The model under review builds one solid part; all positions refer to its coordinate system, in mm. Face numbers are marked on the shaded views. A direction names the side the tool comes from. Round coordinates to 2 decimals unless told otherwise and drop trailing zeros. Order: outer loops, then holes, each group sorted by start corner. A loop starts at its lowest first (then second) coordinate and runs counter-clockwise, first axis right, second up. Notation, with made-up numbers: M -4.5,-25.75 L 0.5,-25.75 A18 cw 0.5,5.25 Z; hole C -10,-6 d5. An arc over 180 degrees is marked long. One line per item, written item: value. Start each with the question number.
from build123d import *

# Parameters (mm, degrees)
SKETCH_1_W      = 15
SKETCH_1_H      = 36
EXTRUDE_1_DEPTH = 29.3
SKETCH_2_R      = 9.975
SKETCH_2_R_2    = 1
EXTRUDE_2_DEPTH = 5.5
EXTRUDE_START   = -19.7
SKETCH_3_W      = 15
SKETCH_3_H      = 6.4
SKETCH_3_R      = 2.1
SKETCH_3_W_2    = 6.4
SKETCH_3_H_2    = 7.5
EXTRUDE_3_DEPTH = 2
SKETCH_4_W      = 6
SKETCH_4_H      = 5
EXTRUDE_4_DEPTH = 4


with BuildPart() as part:
    # 스케치1 → 보스-돌출1 (new body)
    with BuildSketch(Plane.XY):
        Rectangle(SKETCH_1_W, SKETCH_1_H)
    extrude(amount=EXTRUDE_1_DEPTH)

    # 스케치2 → 보스-돌출2 (add)
    with BuildSketch(Plane.XY.offset(29.3)):
        with Locations(Location((0, 6, 0), (0, 0, 221.246533369))):
            Circle(SKETCH_2_R)
        with Locations((0, 13)):
            Circle(SKETCH_2_R_2, mode=Mode.SUBTRACT)
        with Locations(Location((7, 6, 0), (0, 0, 60))):
            Circle(SKETCH_2_R_2, mode=Mode.SUBTRACT)
        with Locations((0, -1)):
            Circle(SKETCH_2_R_2, mode=Mode.SUBTRACT)
        with Locations(Location((-7, 6, 0), (0, 0, 120))):
            Circle(SKETCH_2_R_2, mode=Mode.SUBTRACT)
    extrude(amount=EXTRUDE_2_DEPTH)

    # 스케치3 → 보스-돌출3 (add)
    # profile 1 of 3: a face of its own
    with BuildSketch(Plane(origin=(0, 0, 0), x_dir=(-1, 0, 0), z_dir=(0, 0, -1)).offset(EXTRUDE_START)):
        with Locations((0, -21.2)):
            Rectangle(SKETCH_3_W, SKETCH_3_H)
        with Locations((-3.75, -21.3)):
            Circle(SKETCH_3_R, mode=Mode.SUBTRACT)
        with Locations((3.75, -21.3)):
            Circle(SKETCH_3_R, mode=Mode.SUBTRACT)
    # profile 2 of 3: a face of its own
    with BuildSketch(Plane(origin=(0, 0, 0), x_dir=(-1, 0, 0), z_dir=(0, 0, -1)).offset(EXTRUDE_START)):
        with Locations((-10.7, 9.75)):
            Rectangle(SKETCH_3_W_2, SKETCH_3_H_2)
        with Locations((-10.8, 9.75)):
            Circle(SKETCH_3_R, mode=Mode.SUBTRACT)
    # profile 3 of 3: a face of its own
    with BuildSketch(Plane(origin=(0, 0, 0), x_dir=(-1, 0, 0), z_dir=(0, 0, -1)).offset(EXTRUDE_START)):
        with Locations((10.7, 9.75)):
            Rectangle(SKETCH_3_W_2, SKETCH_3_H_2)
        with Locations((10.8, 9.75)):
            Circle(SKETCH_3_R, mode=Mode.SUBTRACT)
    extrude(amount=-EXTRUDE_3_DEPTH)

    # 스케치4 → 보스-돌출4 (add)
    with BuildSketch(Plane.XZ.offset(18)):
        with Locations((0, 2.5)):
            Rectangle(SKETCH_4_W, SKETCH_4_H)
    extrude(amount=EXTRUDE_4_DEPTH)


solid = part.part
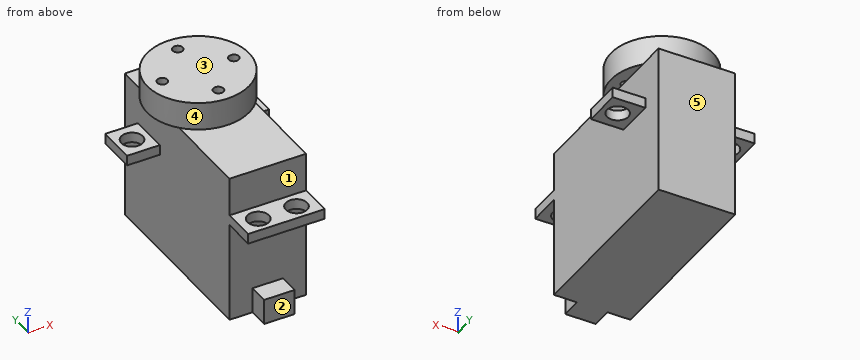
Item 1: Wall thickness on L1, parallel to Y at x = 0, z = 30.95 (3 decimals); L2, parallel to X at y = -14, z = 7.5; L3, parallel to Z at x = -6.75, y = -12: over which ranges is each line inside the solid? List them lowest first.
Item 2: Consider section D-D, the plane z = 3. Give the boundary of the cut face in (x, y).
Item 3: Consider section C-C, the plane y = 9.75. Give the boundary of the cut face in (x, z).
Item 4: Machinability: for the marked faces 1, 2, 3, 4 and 5, which of the approach directions +Z, -Z, +X, -X, +Y, -Y give a long, thin tool a straight path to every point of the face, cutting with its end or side? Answer none if there is none.
Item 5: Consider section B-B, the plane x = 10.8. Give the boundary of the cut face in (y, z), then the cut area to 3 significant figures.
Item 6: Consider section A-A, the plane z = 20.5. Give the boundary of the cut face in (x, y), then the cut area to 3 significant figures.
Item 7: Clearance check with flat-ended pins moving along their axes: P1, Ø3.5, axis at x = 10.8, y = 9.75, coming from the +Z side; P2, Ø1.9, axis at x = 0.5, y = -20, coming from the +Z side; P3, Ø5, axis at x = 7, z = 27, coming from the -Y side; P4, Ø4.5, axis at x = 3, y = -10, coming from the +Z side. State where each tip first meets the part, or that it passes through.
Computed:
1. L1: y = -3.975 to -2, 0 to 12, 14 to 15.975
1. L2: x = -7.5 to 7.5
1. L3: z = 0 to 29.3
2. outline: M -7.5,-18 L -3,-18 L -3,-22 L 3,-22 L 3,-18 L 7.5,-18 L 7.5,18 L -7.5,18 Z
3. outline: M -13.9,19.7 L -12.9,19.7 L -12.9,21.7 L -13.9,21.7 Z; M -9.24,29.3 L -7.5,29.3 L -7.5,21.7 L -8.7,21.7 L -8.7,19.7 L -7.5,19.7 L -7.5,0 L 7.5,0 L 7.5,19.7 L 8.7,19.7 L 8.7,21.7 L 7.5,21.7 L 7.5,29.3 L 9.24,29.3 L 9.24,34.8 L -9.24,34.8 Z; M 12.9,19.7 L 13.9,19.7 L 13.9,21.7 L 12.9,21.7 Z
4. face 1: +Z, +X, -X, -Y
4. face 2: -Z, +X, -X, -Y
4. face 3: +Z, +X, -X, +Y, -Y
4. face 4: +Z
4. face 5: +Z, -Z, +X, -X, +Y
5. outline: M 6,19.7 L 7.65,19.7 L 7.65,21.7 L 6,21.7 Z; M 11.85,19.7 L 13.5,19.7 L 13.5,21.7 L 11.85,21.7 Z
5. area: 6.60 mm^2
6. outline: M -13.9,6 L -7.5,6 L -7.5,-24.4 L 7.5,-24.4 L 7.5,6 L 13.9,6 L 13.9,13.5 L 7.5,13.5 L 7.5,18 L -7.5,18 L -7.5,13.5 L -13.9,13.5 Z; hole C -10.8,9.75 d4.2; hole C -3.75,-21.3 d4.2; hole C 3.75,-21.3 d4.2; hole C 10.8,9.75 d4.2
6. area: 677 mm^2
7. P1: stops at z = 34.8
7. P2: stops at z = 21.7
7. P3: stops at y = -18
7. P4: stops at z = 29.3
